from build123d import *

# Parameters (mm, degrees)
SKETCH1_W           = 150
SKETCH1_H           = 120
BOSS_EXTRUDE1_DEPTH = 25
SHELL1_T            = -2


with BuildPart() as part:
    # Sketch1 → Boss-Extrude1 (new, symmetric)
    with BuildSketch(Plane.XY):
        Rectangle(SKETCH1_W, SKETCH1_H)
    extrude(amount=BOSS_EXTRUDE1_DEPTH, both=True)

    # Shell1
    shell1_openings = [part.faces().sort_by_distance(p)[0] for p in [
        (0, 0, 25),
    ]]
    offset(amount=SHELL1_T, openings=shell1_openings, kind=Kind.INTERSECTION)


solid = part.part
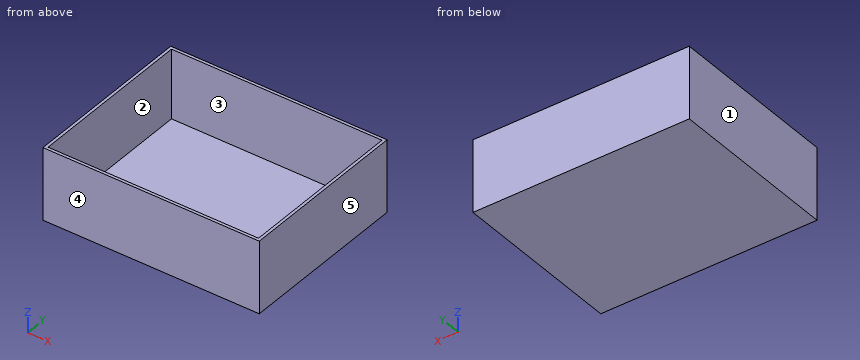
Read the model definition and answer for the solid it produces. Units are mm, in the model's axes. Face numbers are marked on the shaded views. A direction names the side the tool comes from. Round coordinates to 2 decimals unless told otherwise and drop trailing zeros. Write each loop counter-clockwise with the first axis right and the second up, starting at its lowest first coordinate (ties: lowest second). Pieces come first, ordered by that corner, then holes.
1. The part is cut by section C-C, the plane z = -12. Determine the outline of the cut face in (x, y).
2. Straight lines are drawn through the part: L1, parallel to Y at x = 37.5, z = -22; L2, parallel to X at y = -53, z = 3; L3, parallel to Z at x = 44.5, y = 7. For each, find the intervals that lie inside material, in ascending order.
3. The part is cut by section A-A, the plane y = -23.5. Determine the outline of the cut face in (x, z), then the cut area to 3 significant figures.
4. Given pin 1 Ø12 at (x, y) = (-21, -25) entering from +Z, flat-ended and moving along its own axis, determine where the tip first touches the part or whether it passes through.
5. Determine the mould class of the marked faces 3, 4 and 5 for opening direction X: pulls with the +X half, pulls with the -X half, needs draft (parallel to the pull), parting line crosses it, or undercut.
6. Which of the six approach directions +Z, -Z, +X, -X, +Y, -Y give full straight-line access (tool end or side, diameter ignored) to the marked faces 1 and 2?
7. The part is cut by section B-B, the plane x = -41. Determine the outline of the cut face in (y, z), then the cut area to 3 significant figures.
Values:
1. outline: (-75, -60) - (75, -60) - (75, 60) - (-75, 60) - close; hole (-73, -58) - (73, -58) - (73, 58) - (-73, 58) - close
2. L1: y = -60 to -58, 58 to 60
2. L2: x = -75 to -73, 73 to 75
2. L3: z = -25 to -23
3. outline: (-75, -25) - (75, -25) - (75, 25) - (73, 25) - (73, -23) - (-73, -23) - (-73, 25) - (-75, 25) - close
3. area: 492 mm2
4. pin 1: stops at z = -23
5. face 3: undercut
5. face 4: needs draft
5. face 5: pulls with the +X half
6. face 1: +Z, -Z, -X, +Y, -Y
6. face 2: +Z
7. outline: (-60, -25) - (60, -25) - (60, 25) - (58, 25) - (58, -23) - (-58, -23) - (-58, 25) - (-60, 25) - close
7. area: 432 mm2
